from build123d import *

# Parameters (mm, degrees)
F0_W     = 97.5
F0_H     = 5
F0_W_2   = 5
F0_H_2   = 97.5
F1_DEPTH = 1


with BuildPart() as f1:
    # F0 (on Top) → F1 (new body)
    with BuildSketch(Plane.XY):
        with Locations((-51.25, 0)):
            Rectangle(F0_W, F0_H)
        with Locations((0, 51.25)):
            Rectangle(F0_W_2, F0_H_2)
        Rectangle(F0_W_2, F0_H)
        with Locations((51.25, 0)):
            Rectangle(F0_W, F0_H)
        with Locations((0, -51.25)):
            Rectangle(F0_W_2, F0_H_2)
    extrude(amount=F1_DEPTH)


solid = f1.part
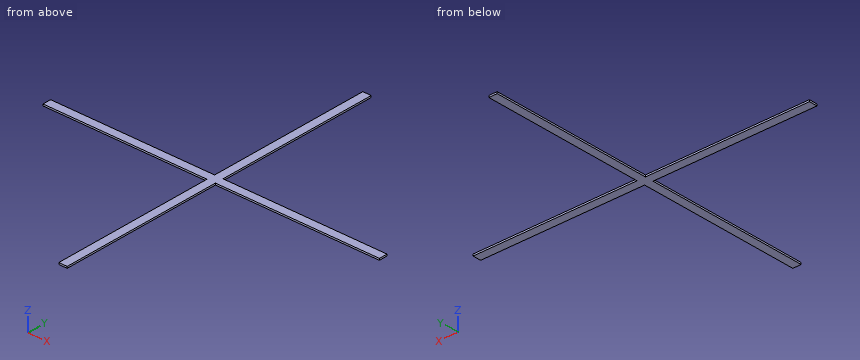
For this review, take the finished solid that the model builds, in its own axes (mm). Coordinates: 2 decimals unless noted, no trailing zeros. Loops run counter-clockwise (first coordinate to the right, second up) from the corner with the lowest first, then second, coordinate; pieces in that order, holes last. Notation, with made-up numbers: (49.5, 42.5) - (103.5, 42.5) arc R23 cw to (103.5, 57.5) - close; hole circle Ø4 at (12.5, 14.25). An arc over 180 degrees is marked (long way). Use a Markdown table: item, result. Add a question column.
Item 1: We need section B-B (x = -54.5). Give the boundary of the cut face in (y, z).
Item 2: Insertion check: pin 1 Ø0.5 at (y, z) = (-59, 0.5) entering from +X; pin 2 Ø0.5 at (x, z) = (-27.5, 0.5) entering from -Y. Each pin has a flat end and moves straight along its axis. Give the tip position at first contact, or say it passes through.
Item 3: For line 1 (Y direction, x = 87, z = 0.6), list the stretches that pass through material, from the lowest coordinate up.
Item 4: We need section A-A (z = 0.7). Give the boundary of the cut face in (x, y), and give its area (4 significant figures).
Results list:
| question | item | result |
|---|---|---|
| 1 | outline | (-2.5, 0) - (2.5, 0) - (2.5, 1) - (-2.5, 1) - close |
| 2 | pin 1 | stops at x = 2.5 |
| 2 | pin 2 | stops at y = -2.5 |
| 3 | line 1 | y = -2.5 to 2.5 |
| 4 | outline | (-100, -2.5) - (-2.5, -2.5) - (-2.5, -100) - (2.5, -100) - (2.5, -2.5) - (100, -2.5) - (100, 2.5) - (2.5, 2.5) - (2.5, 100) - (-2.5, 100) - (-2.5, 2.5) - (-100, 2.5) - close |
| 4 | area | 1,975 mm^2 |
